Source: CAD feature listing. Evaluate the final solid. Frame: model axes, mm. Face numbers are marked on the shaded views. A direction names the side the tool comes from. Round coordinates to 2 decimals unless told otherwise and drop trailing zeros. Loops run counter-clockwise (first coordinate to the right, second up) from the corner with the lowest first, then second, coordinate; pieces in that order, holes last. Notation, with made-up numbers: (86, 18) - (105, 18) arc R27 ccw to (105, 46) - close; hole circle Ø3 at (54.25, -9.75). An arc over 180 degrees is marked (long way). One line per question, with ' | ' between items.
Autodesk Inventor part; units mm, degrees
ref_plane "YZ Plane" through (0, 0, 0) normal (1, 0, 0) x (0, 1, 0)
ref_plane "XZ Plane" through (0, 0, 0) normal (0, 1, 0) x (-1, 0, 0)
ref_plane "XY Plane" through (0, 0, 0) normal (0, 0, 1) x (1, 0, 0)
sketch "Sketch1" plane through (0, 0, 0) normal (0, 0, 1) x (1, 0, 0)
  circle A0 centre (0, 0) radius 1.5
  dimension "d0" = 3
extrude "Extrusion1" add sketch "Sketch1" along normal blind 30
ref_plane "Work Plane1" through (0, 0, 23.5) normal (0, 0, 1) x (1, 0, 0)
ref_plane "Work Plane2" through (0, 0, 6.5) normal (0, 0, -1) x (-1, 0, 0)
sketch "Sketch2" plane through (0, 0, 23.5) normal (0, 0, 1) x (1, 0, 0)
  circle A0 centre (0, 0) radius 1.5
  line L0 (1, 0) -> (-1, 0)
  line L1 (-1, 0) -> (-1, 27.5)
  line L2 (-1, 27.5) -> (1, 27.5)
  line L3 (1, 27.5) -> (1, 0)
  dimension "d7" = 27.5
  dimension "d13" = 1
extrude "Extrusion2" add sketch "Sketch2" against normal up to surface (17 mm away) contours L3 L0 L1 A0 | A0 L1 L2 L3 picked at (0, 0.5)
sketch "Sketch3" plane through (1, 1.118, 23.5) normal (1, 0, 0) x (0, 0, -1)
  line L0 (17, 0) -> (17, 26.382)
  line L1 (0, 26.382) -> (17, 26.382)
  line L2 (0, 26.382) -> (0, 0)
  line L3 (17, 0) -> (0, 0)
  line L4 (0, 26.382) -> (-6.5, 26.382)
  line L5 (-6.5, 26.382) -> (-6.5, 5.882)
  line L6 (-6.5, 5.882) -> (0, 5.882)
  line L7 (0, 5.882) -> (0, 26.382)
  line L8 (17, 0) -> (17, 26.382)
  line L9 (17, 26.382) -> (23.5, 26.382)
  line L10 (23.5, 26.382) -> (23.5, 5.882)
  line L11 (23.5, 5.882) -> (17, 5.882)
  line L12 (17, 5.882) -> (17, 26.382)
  line L13 (23.5, -2.618) -> (23.5, 0.382)
  line L14 (-6.5, 0.382) -> (-6.5, -2.618)
  line L15 (0, 0) -> (17, 0)
  line L16 (17, 0) -> (17, 0)
  line L17 (17, 0) -> (0, 0)
  line L18 (0, 0) -> (0, 0)
  point P0 (23.5, -1.118)
  point P1 (20.25, 5.882)
  point P2 (-3.25, 5.882)
  point P3 (23.5, -1.118)
  point P4 (23.5, 16.132)
  point P5 (-6.5, 16.132)
  point P6 (-6.5, -1.118)
  dimension "d10" = 5.5
extrude "Extrusion3" add sketch "Sketch3" against normal up to surface (2 mm away) contours L0 L9 L10 L11 | L6 L5 L4 L2
sketch "Sketch5" plane through (-1, 1.118, 6.5) normal (-1, 0, 0) x (0, 0, 1)
  line L0 (17, 0) -> (0, 0)
  line L1 (17, 0) -> (17, 5.882)
  line L2 (23.5, 5.882) -> (17, 5.882)
  line L3 (23.5, 26.382) -> (23.5, 5.882)
  line L4 (23.5, 26.382) -> (-6.5, 26.382)
  line L5 (-6.5, 5.882) -> (-6.5, 26.382)
  line L6 (0, 5.882) -> (-6.5, 5.882)
  line L7 (0, 5.882) -> (0, 0)
  line L8 (23.5, 5.882) -> (17, 5.882)
  line L9 (23.5, 26.382) -> (-6.5, 26.382)
  line L10 (23.5, 5.882) -> (20.5, 5.882)
  line L11 (20.5, 5.882) -> (20.5, 26.382)
  line L12 (20.5, 26.382) -> (23.5, 26.382)
  line L13 (23.5, 26.382) -> (23.5, 5.882)
  line L14 (0, 5.882) -> (-6.5, 5.882)
  line L15 (-6.5, 26.382) -> (-1.1, 26.382)
  line L16 (-1.1, 26.382) -> (-1.1, 5.882)
  line L17 (-1.1, 5.882) -> (-6.5, 5.882)
  line L18 (-6.5, 5.882) -> (-6.5, 26.382)
  point P0 (-6.5, -1.118)
  dimension "d16" = 3
  dimension "d17" = 5.4
extrude "Extrusion5" add sketch "Sketch5" along normal blind 1.26 contours L11 L4 L3 L2 | L6 L5 L4 L16
properties part number "gpsDoor"
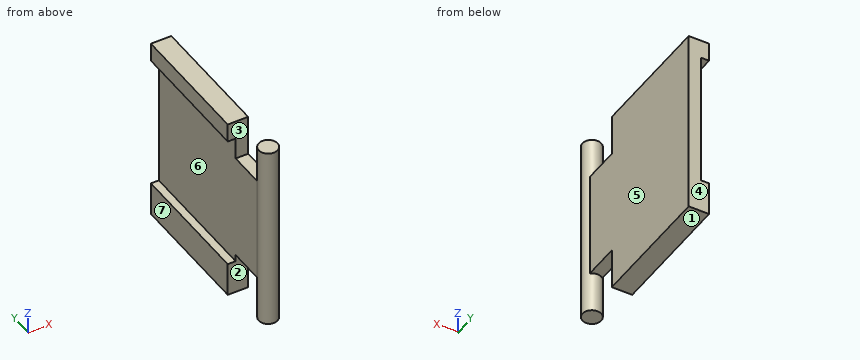
1. Contact query for flat-ended pins moving along their axis: P1, Ø0.6, axis at x = -0.5, y = 3, coming from the -Z side; P2, Ø1, axis at x = 0.5, y = 5, coming from the +Z side; P3, Ø1, axis at x = -0.5, z = 2, coming from the -Y side; P4, Ø10, axis at y = 7.5, z = 11.5, coming from the +X side. Output: stop coordinate, or through.
Worked out:
P1: stops at z = 6.5 | P2: stops at z = 23.5 | P3: stops at y = -1.5 | P4: stops at x = 1
2. Section query A-A, the plane z = 26. Return loops of the section in (x, y), plus the area to 3 significant figures.
Worked out:
outline: circle Ø3 at (0, 0); (-1, 7) - (1, 7) - (1, 27.5) - (-1, 27.5) - close | area: 48.1 mm2
3. Material intervals for probe 1 along Z at (x, y) = (-1.85, 13.25); probe 2 along X at (y, z) = (23, 21); probe 3 along X at (y, z) = (17.5, 27.5), sorted ascending.
Worked out:
probe 1: z = 0 to 5.4, 27 to 30 | probe 2: x = -1 to 1 | probe 3: x = -2.26 to 1
4. Access query for the marked faces 5, 6 and 7. Directions: +Z, -Z, +X, -X, +Y, -Y. A direction counts if a zero-diameter tool reaches every point of the face in a straight line with its end or side. Return the directions, or none.
Worked out:
face 5: +Z, -Z, +X, +Y | face 6: -X, +Y | face 7: +Z, -Z, -X, +Y, -Y
5. Section query B-B, the plane y = 14.5. Return loops of the section in (x, z), plus the area to 3 significant figures.
Worked out:
outline: (-2.26, 0) - (1, 0) - (1, 30) - (-2.26, 30) - (-2.26, 27) - (-1, 27) - (-1, 5.4) - (-2.26, 5.4) - close | area: 70.6 mm2
6. Mould query, pull axis Y, two halves, no side actions, for the marked faces 1, 2, 3 and 4. Classes: released by +Y, released by -Y, zero draft, split by the parting line, or undercut.
Worked out:
face 1: zero draft | face 2: undercut | face 3: undercut | face 4: released by +Y
7. Section query C-C, the plane x = 0. Return loops of the section in (y, z).
Worked out:
outline: (-1.5, 0) - (1.5, 0) - (1.5, 6.5) - (7, 6.5) - (7, 0) - (27.5, 0) - (27.5, 30) - (7, 30) - (7, 23.5) - (1.5, 23.5) - (1.5, 30) - (-1.5, 30) - close
8. Section query D-D, the plane z = 15.75. Return loops of the section in (x, y), plus the area to 3 significant figures.
Worked out:
outline: (-1, 1.12) arc R1.5 ccw (long way) to (1, 1.12) - (1, 27.5) - (-1, 27.5) - close | area: 59.3 mm2
